```python
from build123d import *

# Parameters (mm, degrees)
BOSS_EXTRUDE2_DEPTH = 6.35
SKETCH40_R          = 2
CUT_EXTRUDE1_DEPTH  = 6.35
SKETCH41_R          = 2
CUT_EXTRUDE2_DEPTH  = 6.35


with BuildPart() as part:
    # Sketch1 → Boss-Extrude2 (new body)
    with BuildSketch(Plane(origin=(0, 0, 0), x_dir=(1, 0, 0), z_dir=(0, 1, 0))):
        with BuildLine():
            Line((152.4, -101.6), (152.4, -50.8))
            Line((152.4, -50.8), (190.076195248, -12.7))
            ThreePointArc((190.076195248, -12.7), (190.5, 0), (190.076195248, 12.7))
            Line((190.076195248, 12.7), (152.4, 50.8))
            Line((152.4, 50.8), (152.4, 101.6))
            Line((152.4, 101.6), (157.687433266, 106.887433266))
            ThreePointArc((157.687433266, 106.887433266), (155.08800922, 110.62531083), (152.4, 114.3))
            ThreePointArc((152.4, 114.3), (129.141828926, 140.045128518), (101.6, 161.144934764))
            Line((101.6, 161.144934764), (101.6, 135.744934764))
            Line((101.6, 135.744934764), (124.436872293, 135.744934764))
            ThreePointArc((124.436872293, 135.744934764), (135.756435031, 124.424325787), (146.05, 112.163363002))
            Line((146.05, 112.163363002), (146.05, 6.35))
            Line((146.05, 6.35), (133.35, 6.35))
            Line((133.35, 6.35), (133.35, -6.35))
            Line((133.35, -6.35), (146.05, -6.35))
            Line((146.05, -6.35), (146.05, -112.163363002))
            ThreePointArc((146.05, -112.163363002), (135.756435031, -124.424325787), (124.436872293, -135.744934764))
            Line((124.436872293, -135.744934764), (101.6, -135.744934764))
            Line((101.6, -135.744934764), (101.6, -161.144934764))
            ThreePointArc((101.6, -161.144934764), (129.141828926, -140.045128518), (152.4, -114.3))
            ThreePointArc((152.4, -114.3), (155.08800922, -110.62531083), (157.687433266, -106.887433266))
            Line((157.687433266, -106.887433266), (152.4, -101.6))
        make_face()
    extrude(amount=BOSS_EXTRUDE2_DEPTH)

    # Sketch40 → Cut-Extrude1 (cut)
    with BuildSketch(Plane(origin=(0, 6.35, 0), x_dir=(1, 0, 0), z_dir=(0, 1, 0))):
        with Locations((139.7, 0)):
            Circle(SKETCH40_R)
    extrude(amount=-CUT_EXTRUDE1_DEPTH, mode=Mode.SUBTRACT)

    # Sketch41 → Cut-Extrude2 (cut)
    with BuildSketch(Plane(origin=(0, 6.35, 0), x_dir=(1, 0, 0), z_dir=(0, 1, 0))):
        with Locations((114.080655546, 142.381475202)):
            Circle(SKETCH41_R)
        with Locations((114.080655546, -142.381475202)):
            Circle(SKETCH41_R)
    extrude(amount=-CUT_EXTRUDE2_DEPTH, mode=Mode.SUBTRACT)


solid = part.part
```
Read the model definition and answer for the solid it produces. Units are mm, in the model's axes. A direction names the side the tool comes from. Round coordinates to 2 decimals unless told otherwise and drop trailing zeros. Write each loop counter-clockwise with the first axis right and the second up, starting at its lowest first coordinate (ties: lowest second). Pieces come first, ordered by that corner, then holes. Notation, with made-up numbers: (-15, -11) - (-11, -11) arc R14 cw to (-11, 10) - close; hole circle Ø11 at (85, 51). An arc over 180 degrees is marked (long way). Use CSV: the item, a comma, the result in double quotes.
Q1. Straight lines are drawn through the part: line 1 along X through (y, z) = (2.75, 0); line 2 along Z through (x, y) = (135, 4.5); line 3 along Z through (x, y) = (139.7, 2.75). For each, find the intervals that lie inside material, in ascending order.
Values:
line 1,"x = 133.35 to 137.7, 141.7 to 190.5"
line 2,"z = -134.41 to -125.24, -6.35 to 6.35, 125.24 to 134.41"
line 3,"z = -129.52 to -119.98, -6.35 to -2, 2 to 6.35, 119.98 to 129.52"
Q2. A tool of negligible diameter and unlimited length cuts with its end or side. For faces 1 (the cylindrical face through (135.908, 3.131, 124.259)), 2 (the flat face through (152.4, 3, 77)), 3 (the flat face through (152, 0, -1)), from which of +Z, -Z, +X, -X, +Y, -Y can it reach the whole face along a straight path? Write none if from no direction.
Values:
face 1,"-X, +Y, -Y"
face 2,"+X, +Y, -Y"
face 3,"+Z, -Z, +X, -X, -Y"
Q3. Find section B-B, the plane z = 67. Write down the section's boundary in (x, y), then the cut area to 3 significant figures.
Values:
outline,"(146.05, 0) - (152.4, 0) - (152.4, 6.35) - (146.05, 6.35) - close"
area,"40.3 mm²"
Q4. Each of these flat-tipped pins is pushed along its axis until it touches: pin 1 Ø1.9 at (y, z) = (4, 49.5) entering from -X; pin 2 Ø3 at (x, y) = (138.5, 3) entering from -Z; pin 3 Ø4.5 at (x, z) = (114.08, -142.38) entering from -Y; pin 4 Ø1.9 at (x, y) = (115, 4) entering from -Z. Where does it stop, or does it pass through?
Values:
pin 1,"stops at x = 146.05"
pin 2,"stops at z = -132.37"
pin 3,"stops at y = 0"
pin 4,"stops at z = -152.59"
Q5. Find section A-A, the plane y = 2.25. Write down the section's boundary in (x, z), then the cut area to 3 significant figures.
Values:
outline,"(101.6, -161.14) arc R190.5 ccw to (157.69, -106.89) - (152.4, -101.6) - (152.4, -50.8) - (190.08, -12.7) arc R190.5 ccw to (190.08, 12.7) - (152.4, 50.8) - (152.4, 101.6) - (157.69, 106.89) arc R190.5 ccw to (101.6, 161.14) - (101.6, 135.74) - (124.44, 135.74) arc R184.15 cw to (146.05, 112.16) - (146.05, 6.35) - (133.35, 6.35) - (133.35, -6.35) - (146.05, -6.35) - (146.05, -112.16) arc R184.15 cw to (124.44, -135.74) - (101.6, -135.74) - close; hole circle Ø4 at (114.08, -142.38); hole circle Ø4 at (114.08, 142.38); hole circle Ø4 at (139.7, 0)"
area,"5,290 mm²"
Q6. Find section C-C, the plane x = 161.5. Write down the section's boundary in (y, z), then the cut area to 3 significant figures.
Values:
outline,"(0, -41.6) - (6.35, -41.6) - (6.35, 41.6) - (0, 41.6) - close"
area,"528 mm²"
